Can you work these out from the drawing? Everything is in mm from the part's minimum corner. A direction names the side the tool comes from. Coordinates: 2 decimals unless noted, no trailing zeros. Loops run counter-clockwise (first coordinate to the right, second up) from the corner with the lowest first, then second, coordinate; pieces in that order, holes last. Notation, with made-up numbers: (50.5, 3) -> (87.5, 3) arc R29 ccw to (87.5, 25) -> close; hole circle Ø9 at (26, 77). An arc over 180 degrees is marked (long way). Put each result on its own line as item: value. Start each with the question number.
Item 1: If we section it at C-C on y = 12: Please give me the cut outline in (x, z), plus the area to 3 significant figures.
Item 2: Will these pins go through, and if not, where does the flat tip stop? P1, Ø2, axis at y = 3, z = 1, coming from the +X side; P2, Ø4, axis at x = 9.5, z = 2.5, coming from the -Y side.
Item 3: If we section it at A-A on z = 6.75: Please give me the cut outline in (x, y).
Item 4: If we section it at B-B on x = 1.5: Please give me the cut outline in (y, z).
Item 5: Please list where these lines run through material, in increasing order: L1, parallel to Y at x = 3, z = 5; L2, parallel to Y at x = 9.5, z = 1; L3, parallel to X at y = 3, z = 4. Write a range as from..to.
Item 6: If we section it at D-D on x = 10: Please give me the cut outline in (y, z).
Item 7: We'd pull the mould along Y, two halves only. Please class the marked faces 3, 4 and 5: pulls with the +Y half, pulls with the -Y half, needs draft (parallel to the pull), parting line crosses it, or undercut.
Item 8: For the marked faces 1 and 2, which set-ups out of +Z, -Z, +X, -X, +Y, -Y let a thin tool reach every point of the face, with its end or its side?
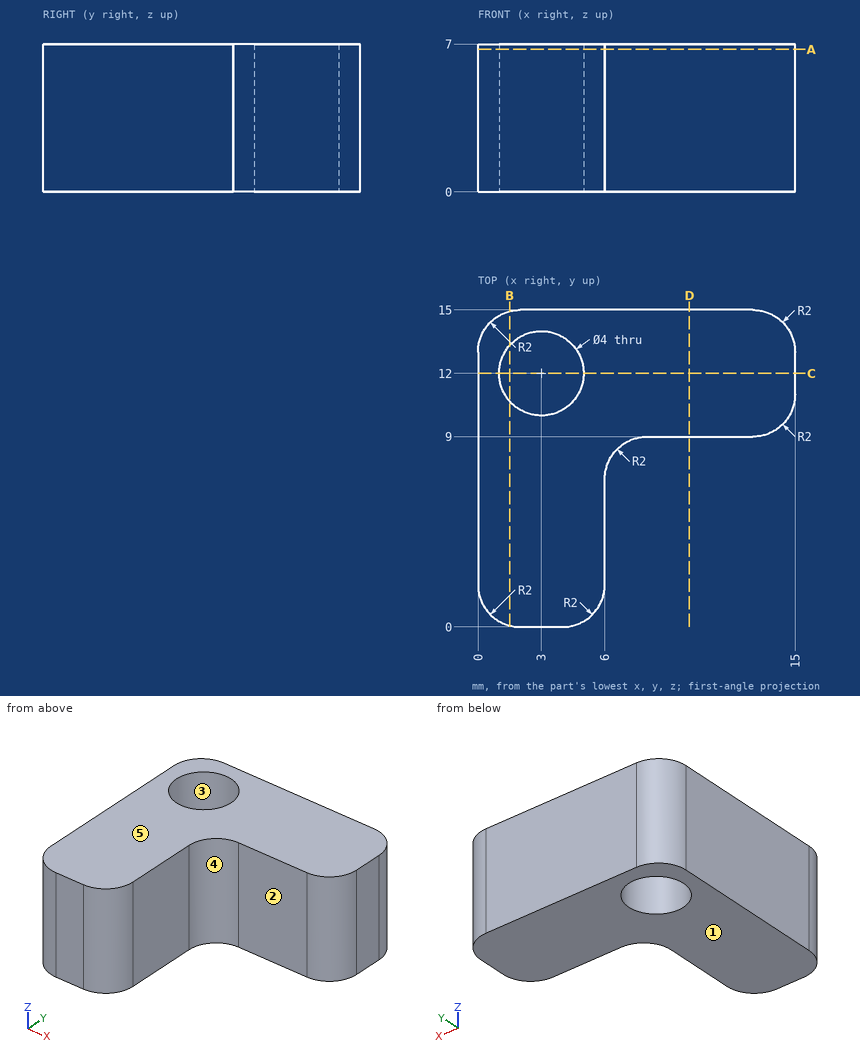
Solutions:
1. outline: (0, 0) -> (1, 0) -> (1, 7) -> (0, 7) -> close; (5, 0) -> (15, 0) -> (15, 7) -> (5, 7) -> close
1. area: 77.0 mm^2
2. P1: x = 6
2. P2: y = 8.94
3. outline: (0, 2) arc R2 ccw to (2, 0) -> (4, 0) arc R2 ccw to (6, 2) -> (6, 7) arc R2 cw to (8, 9) -> (13, 9) arc R2 ccw to (15, 11) -> (15, 13) arc R2 ccw to (13, 15) -> (2, 15) arc R2 ccw to (0, 13) -> close; hole circle Ø4 at (3, 12)
4. outline: (0.06, 0) -> (10.68, 0) -> (10.68, 7) -> (0.06, 7) -> close; (13.32, 0) -> (14.94, 0) -> (14.94, 7) -> (13.32, 7) -> close
5. L1: 0..10, 14..15
5. L2: 9..15
5. L3: 0..6
6. outline: (9, 0) -> (15, 0) -> (15, 7) -> (9, 7) -> close
7. face 3: undercut
7. face 4: pulls with the -Y half
7. face 5: needs draft
8. face 1: -Z, +X, -X, +Y, -Y
8. face 2: +Z, -Z, +X, -Y
